Autodesk Inventor part; units mm, degrees
ref_plane "Work Plane1" through (0, 2.54, 44.45) normal (0, 1, 0) x (-1, 0, 0)
ref_plane "YZ Plane" through (0, 0, 0) normal (1, 0, 0) x (0, 1, 0)
ref_plane "XZ Plane" through (0, 0, 0) normal (0, 1, 0) x (-1, 0, 0)
sketch "Sketch1" plane through (0, 0, 0) normal (0, 0, 1) x (1, 0, 0)
  circle A0 centre (0, 0) radius 2.54
  dimension "d0" = 5.08
extrude "Extrusion1" add sketch "Sketch1" along normal blind 44.45
sketch "Sketch2" plane through (0, 0, 44.45) normal (0, 0, 1) x (1, 0, 0)
  circle A0 centre (0, 0) radius 2.54
  point P0 (0, 2.54)
ref_plane "Work Plane1" through (0, 2.54, 44.45) normal (0, 1, 0) x (-1, 0, 0)
sketch "Sketch3" plane through (0, 2.54, 44.45) normal (0, 1, 0) x (-1, 0, 0)
  circle A0 centre (0, -39.37) radius 2.54
  circle A1 centre (0, -5.08) radius 2.54
  line L0 (2.54, 0) -> (-2.54, 0)
  point P0 (0, -44.45)
  dimension "d4" = 5.08
  dimension "d6" = 5.08
  dimension "d7" = 5.08
  dimension "d8" = 5.08
extrude "Extrusion2" add sketch "Sketch3" along normal blind 12.7 and the other way blind 2.54
sketch "Sketch4" plane through (0, 15.24, 39.37) normal (0, 1, 0) x (1, 0, 0)
  circle A0 centre (0, 0) radius 2.54
  line L0 (0, 0) -> (0, 34.29) construction
  line L1 (0, 17.145) -> (4.1545, 17.145) construction
  point P0 (0, 39.37)
  dimension "d14" = 34.29
revolve "Revolution1" add sketch "Sketch4" angle 180 about axis through (0, 15.24, 22.225) along (-1, 0, 0)
properties part number "0D" material "Stainless Steel"
Part model, mm, in its own coordinate system. Round coordinates to 2 decimals unless told otherwise and drop trailing zeros. Loops run counter-clockwise (first coordinate to the right, second up) from the corner with the lowest first, then second, coordinate; pieces in that order, holes last.
1. Slice it at C-C (y = 2). Give the cut face in (x, z), and give its area (3 significant figures).
Solutions:
outline: (-1.57, 0) - (1.57, 0) - (1.57, 3.08) arc R2.54 ccw to (1.57, 7.08) - (1.57, 37.37) arc R2.54 ccw to (1.57, 41.37) - (1.57, 44.45) - (-1.57, 44.45) - (-1.57, 41.37) arc R2.54 ccw to (-1.57, 37.37) - (-1.57, 7.08) arc R2.54 ccw to (-1.57, 3.08) - close
area: 150 mm2
2. Slice it at B-B (y = 13). Give the cut face in (x, z), and give its area (3 significant figures).
Solutions:
outline: circle Ø5.08 at (0, 5.08); circle Ø5.08 at (0, 39.37)
area: 40.5 mm2
3. Slice it at A-A (x = 0). Give the cut face in (y, z) (3 decimals), and give its area (3 significant figures).
Solutions:
outline: (-2.54, 0) - (2.54, 0) - (2.54, 2.54) - (15.24, 2.54) arc R19.685 ccw to (15.24, 41.91) - (2.54, 41.91) - (2.54, 44.45) - (-2.54, 44.45) - close; hole (2.54, 7.62) - (15.24, 7.62) arc R14.605 ccw to (15.24, 36.83) - (2.54, 36.83) - close
area: 628 mm2
4. Drill centre lines: line 1 along Z through (x, y) = (-1.85, 9); line 2 along Z through (x, y) = (-2.2, 12); line 3 along Y through (x, z) = (0.2, 32.5). Where is each one in solid material? Low to high.
Solutions:
line 1: z = 3.34 to 6.82, 37.63 to 41.11
line 2: z = 3.81 to 6.35, 38.1 to 40.64
line 3: y = -2.53 to 2.53, 25.63 to 32.02
5. Flat gauge pins, fed straight in: pin 1 (1.5 mm diameter, centred on x = 2, z = 13, fed in from -Y); pin 2 (1 mm diameter, centred on x = 0, y = 25.5, fed in from -Z). Where does each tip first touch, or does it go through?
Solutions:
pin 1: stops at y = -2.21
pin 2: stops at z = 5.13
6. Two-plate mould, pull along Z, no slides. Class faces 1 (the face through (-0.33, -2.52, 21.91)), 2 (the face through (0, 0, 0)), 3 (the face through (0, 0, 44.45)): pulls with the +Z half, pulls with the -Z half, needs draft (parallel to the pull), parting line crosses it, or undercut.
Solutions:
face 1: undercut
face 2: pulls with the -Z half
face 3: pulls with the +Z half
